Can you work these out from the model? Positions are in its coordinate system, mm. Give positions to 0.01 mm unless a question says otherwise; leave off trailing zeros. Write each loop counter-clockwise with the first axis right and the second up, starting at its lowest first coordinate (ties: lowest second). Pieces come first, ordered by that corner, then holes. Notation, with made-up numbers: (64, 38) - (79, 38) arc R27 ccw to (79, 71) - close; hole circle Ø9 at (47.25, -26). An arc over 180 degrees is marked (long way). Return JSON: item names as keys, results as strings. Group by question number.
from build123d import *

# Parameters (mm, degrees)
SKETCH1_W             = 23
SKETCH1_H             = 23
BOSS_EXTRUDE1_DEPTH   = 2
FILLET1_R             = 2
SKETCH2_R             = 1.6
CUT_EXTRUDE1_DEPTH    = 2
SKETCH3_W             = 10.8
SKETCH3_H             = 2.3
CUT_EXTRUDE2_DEPTH    = 2
SKETCH5_R             = 1.6
BOSS_EXTRUDE2_DEPTH   = 2
BOSS_EXTRUDE2_2_DEPTH = 2
BOSS_EXTRUDE2_3_DEPTH = 2
BOSS_EXTRUDE2_4_DEPTH = 2


with BuildPart() as part:
    # Sketch1 → Boss-Extrude1 (new body)
    with BuildSketch(Plane.XY):
        with Locations((11.5, 11.5)):
            Rectangle(SKETCH1_W, SKETCH1_H)
    extrude(amount=BOSS_EXTRUDE1_DEPTH)

    # Fillet1
    fillet1_edges = [part.edges().sort_by_distance(p)[0] for p in [
        (0, 23, 1),
        (23, 23, 1),
        (23, 0, 1),
        (0, 0, 1),
    ]]
    fillet(fillet1_edges, radius=FILLET1_R)

    # Sketch2 → Cut-Extrude1 (cut)
    with BuildSketch(Plane.XY):
        with Locations((3.5, 19.7)):
            Circle(SKETCH2_R)
        with Locations((19.5, 19.7)):
            Circle(SKETCH2_R)
        with Locations((19.5, 3.5)):
            Circle(SKETCH2_R)
        with Locations((3.5, 3.5)):
            Circle(SKETCH2_R)
        with BuildLine():
            Line((3.5, 17.1), (3.5, 6.1))
            ThreePointArc((3.5, 6.1), (5.338477631, 5.338477631), (6.1, 3.5))
            Line((6.1, 3.5), (16.9, 3.5))
            ThreePointArc((16.9, 3.5), (17.661522369, 5.338477631), (19.5, 6.1))
            Line((19.5, 6.1), (19.5, 17.1))
            ThreePointArc((19.5, 17.1), (17.661522369, 17.861522369), (16.9, 19.7))
            Line((16.9, 19.7), (6.1, 19.7))
            ThreePointArc((6.1, 19.7), (5.338477631, 17.861522369), (3.5, 17.1))
        make_face()
    extrude(amount=CUT_EXTRUDE1_DEPTH, mode=Mode.SUBTRACT)

    # Sketch3 → Cut-Extrude2 (cut)
    with BuildSketch(Plane.XY):
        with Locations((11.5, 20.85)):
            Rectangle(SKETCH3_W, SKETCH3_H)
    extrude(amount=CUT_EXTRUDE2_DEPTH, mode=Mode.SUBTRACT)


with BuildPart() as body_2:
    # Sketch5 → Boss-Extrude2 (new body)
    with BuildSketch(Plane.XY):
        with BuildLine():
            Line((16.9, 23), (21.776453683, 21.561960094))
            Line((21.776453683, 21.561960094), (23, 12.648059803))
            ThreePointArc((23, 12.648059803), (23.313519219, 13.886650017), (24.17856315, 14.826915413))
            Line((24.17856315, 14.826915413), (29.65108056, 18.405475842))
            ThreePointArc((29.65108056, 18.405475842), (30.877170115, 22.033391556), (27.643175365, 24.084329386))
            Line((27.643175365, 24.084329386), (16.9, 23))
        make_face()
        with Locations((27.954482672, 21)):
            Circle(SKETCH5_R, mode=Mode.SUBTRACT)
    extrude(amount=BOSS_EXTRUDE2_DEPTH)


with BuildPart() as body_3:
    # Sketch5 → Boss-Extrude2 2 (new body)
    with BuildSketch(Plane.XY):
        with BuildLine():
            Line((-4.643175365, 24.084329386), (6.1, 23))
            Line((6.1, 23), (1.223546317, 21.561960094))
            Line((1.223546317, 21.561960094), (0, 12.648059803))
            ThreePointArc((0, 12.648059803), (-0.313519219, 13.886650017), (-1.17856315, 14.826915413))
            Line((-1.17856315, 14.826915413), (-6.65108056, 18.405475842))
            ThreePointArc((-6.65108056, 18.405475842), (-7.877170115, 22.033391556), (-4.643175365, 24.084329386))
        make_face()
        with Locations((-4.954482672, 21)):
            Circle(SKETCH5_R, mode=Mode.SUBTRACT)
    extrude(amount=BOSS_EXTRUDE2_2_DEPTH)


with BuildPart() as body_4:
    # Sketch5 → Boss-Extrude2 3 (new body)
    with BuildSketch(Plane.XY):
        with BuildLine():
            Line((16.9, 0), (21.776453683, 1.438039906))
            Line((21.776453683, 1.438039906), (23, 10.351940197))
            ThreePointArc((23, 10.351940197), (23.313519219, 9.113349983), (24.17856315, 8.173084587))
            Line((24.17856315, 8.173084587), (29.65108056, 4.594524158))
            ThreePointArc((29.65108056, 4.594524158), (30.877170115, 0.966608444), (27.643175365, -1.084329386))
            Line((27.643175365, -1.084329386), (16.9, 0))
        make_face()
        with Locations((27.954482672, 2)):
            Circle(SKETCH5_R, mode=Mode.SUBTRACT)
    extrude(amount=BOSS_EXTRUDE2_3_DEPTH)


with BuildPart() as body_5:
    # Sketch5 → Boss-Extrude2 4 (new body)
    with BuildSketch(Plane.XY):
        with BuildLine():
            Line((6.1, 0), (1.223546317, 1.438039906))
            Line((1.223546317, 1.438039906), (0, 10.351940197))
            ThreePointArc((0, 10.351940197), (-0.313519219, 9.113349983), (-1.17856315, 8.173084587))
            Line((-1.17856315, 8.173084587), (-6.65108056, 4.594524158))
            ThreePointArc((-6.65108056, 4.594524158), (-7.877170115, 0.966608444), (-4.643175365, -1.084329386))
            Line((-4.643175365, -1.084329386), (6.1, 0))
        make_face()
        with Locations((-4.954482672, 2)):
            Circle(SKETCH5_R, mode=Mode.SUBTRACT)
    extrude(amount=BOSS_EXTRUDE2_4_DEPTH)

    # Combine1: union part, body 3, body 2, body 4
    add(part.part)
    add(body_3.part)
    add(body_2.part)
    add(body_4.part)


solid = body_5.part
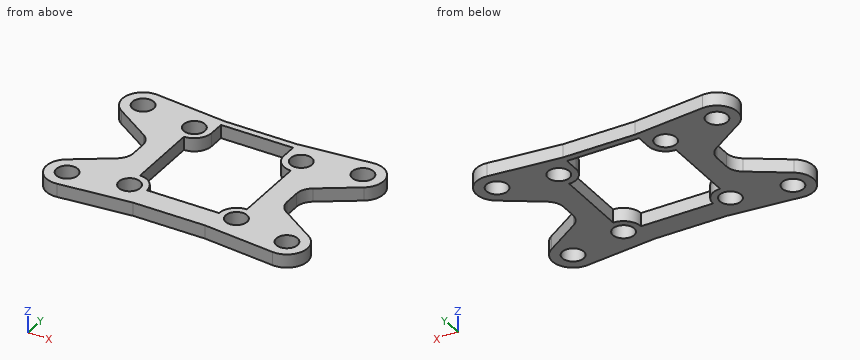
1) Will these pins go through, and if not, where does the flat tip stop? pin 1 Ø5 at (x, y) = (27.95, 21) entering from +Z; pin 2 Ø0.6 at (y, z) = (11, 0.5) entering from +X; pin 3 Ø1 at (x, z) = (10, 0.5) entering from -Y; pin 4 Ø1 at (y, z) = (9.5, 1) entering from -X.
2) Imagine slicing it at D-D, the plane x = 3. Write out the boundary of the cut face in (y, z).
3) Imagine slicing it at B-B, the plane x = 10. Write out the boundary of the cut face in (y, z), and give its area (3 significant figures).
4) I need wall thicknesses on line 1 along Y through (x, z) = (20, 0.9); line 2 along Y through (x, z) = (8, 1.15); line 3 along X through (y, z) = (2.25, 1.55). Which ranges of each line are inside material? Lowest first, please.
5) Imagine slicing it at A-A, the plane y = 11. Write out the boundary of the cut face in (x, z).
6) Imagine slicing it at C-C, the plane y = 2.5. Write out the boundary of the cut face in (x, z), and give its area (3 significant figures).
Resolved:
{
 "1": {"pin 1": "z = 2", "pin 2": "x = 23", "pin 3": "y = 0", "pin 4": "x = -0.38"},
 "2": {"outline": "(-0.31, 0) - (1.98, 0) - (1.98, 2) - (-0.31, 2) - close; (5.02, 0) - (18.18, 0) - (18.18, 2) - (5.02, 2) - close; (21.22, 0) - (23.31, 0) - (23.31, 2) - (21.22, 2) - close"},
 "3": {"outline": "(0, 0) - (3.5, 0) - (3.5, 2) - (0, 2) - close; (22, 0) - (23, 0) - (23, 2) - (22, 2) - close", "area": "9.00 mm^2"},
 "4": {"line 1": "-0.31 to 1.98, 5.02 to 18.18, 21.22 to 23.31", "line 2": "0 to 3.5, 22 to 23", "line 3": "-8.04 to -6.53, -3.37 to 2.5, 4.5 to 18.5, 20.5 to 26.37, 29.53 to 31.04"},
 "5": {"outline": "(0, 0) - (3.5, 0) - (3.5, 2) - (0, 2) - close; (19.5, 0) - (23, 0) - (23, 2) - (19.5, 2) - close"},
 "6": {"outline": "(-8.01, 0) - (-6.47, 0) - (-6.47, 2) - (-8.01, 2) - close; (-3.43, 0) - (2.25, 0) - (2.25, 2) - (-3.43, 2) - close; (4.75, 0) - (18.25, 0) - (18.25, 2) - (4.75, 2) - close; (20.75, 0) - (26.43, 0) - (26.43, 2) - (20.75, 2) - close; (29.47, 0) - (31.01, 0) - (31.01, 2) - (29.47, 2) - close", "area": "55.9 mm^2"}
}
